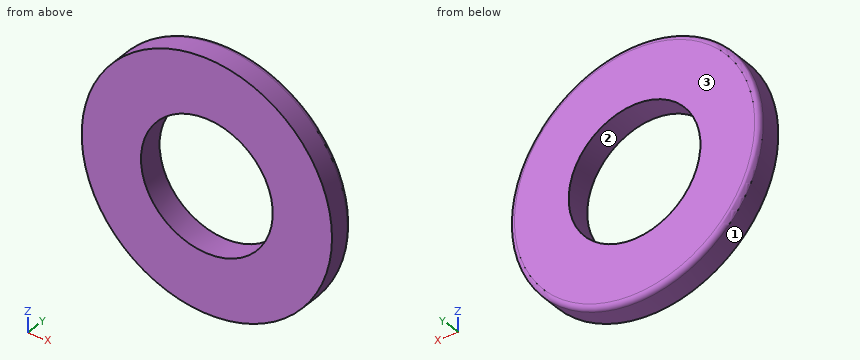
Autodesk Fusion 360 part; units mm, degrees
cylinder "CylindrePrimitive1" add diameter 14.95 height 1.52 placed x (1, 0, 0) y (0, 0, -1) z (0, 1, 0) at (0, 0, 0)
hole "Perçage1" at (0, 1.52, 0) direction (0, -1, 0) diameter 7.87 end through all
fillet "Congé1" radius 0.299 1 edges at (-6.9691, 1.52, 2.7031)
equation "rond_diam = 14.95 mm"
equation "tige_diam = 7.87 mm"
equation "d5 = rond_ep"
equation "rond_ep = 1.52 mm"
equation "d9 = tige_diam"
equation "d12 = rond_diam / 50"
equation "d12 = rond_diam / 50"
Read the model definition and answer for the solid it produces. Units are mm, in the model's axes. Face numbers are marked on the shaded views. Round coordinates to 2 decimals unless told otherwise and drop trailing zeros. Write each loop counter-clockwise with the first axis right and the second up, starting at its lowest first coordinate (ties: lowest second). Pieces come first, ordered by that corner, then holes. Notation, with made-up numbers: (11.25, 15.5) - (22.25, 15.5) arc R14 ccw to (22.25, 19.5) - close; hole circle Ø3 at (28, 76.25). An arc over 180 degrees is marked (long way). Use CSV: the item, a comma, the result in double quotes.
Q1. Straight lines are drawn through the part: line 1 along Z through (x, y) = (0, 1) (3 decimals); line 2 along Z through (x, y) = (2.75, 1.1). For each, find the intervals that lie inside material, in ascending order.
Values:
line 1,"z = -7.475 to -3.935, 3.935 to 7.475"
line 2,"z = -6.95 to -2.81, 2.81 to 6.95"
Q2. Determine the mould class of the marked faces 1, 2 and 3 for opening direction Z: +Z half, -Z half, draft (parallel to the pull), parting line (faces both ways), or undercut.
Values:
face 1,"parting line"
face 2,"undercut"
face 3,"draft"
Q3. Find section B-B, the plane y = 1. Write down the section's boundary in (x, z) (3 decimals), then the cut area to 3 significant figures.
Values:
outline,"circle Ø14.95 at (0, 0); hole circle Ø7.87 at (0, 0)"
area,"127 mm²"
Q4. Find section A-A, the plane z = 0. Write down the section's boundary in (x, y) (3 decimals), then the cut area to 3 significant figures.
Values:
outline,"(-7.475, 0) - (-3.935, 0) - (-3.935, 1.52) - (-7.176, 1.52) arc R0.299 ccw to (-7.475, 1.221) - close; (3.935, 0) - (7.475, 0) - (7.475, 1.221) arc R0.299 ccw to (7.176, 1.52) - (3.935, 1.52) - close"
area,"10.7 mm²"
